from build123d import *

# Parameters (mm, degrees)
SKETCH_1_W      = 20
SKETCH_1_H      = 20
SKETCH_1_R      = 1.6
EXTRUDE_1_DEPTH = 20
FILLET_1_R      = 2


with BuildPart() as part:
    # 草图1 → 凸台-拉伸1 (new body)
    with BuildSketch(Plane(origin=(0, 0, 0), x_dir=(1, 0, 0), z_dir=(0, 1, 0))):
        Rectangle(SKETCH_1_W, SKETCH_1_H)
        Circle(SKETCH_1_R, mode=Mode.SUBTRACT)
    extrude(amount=EXTRUDE_1_DEPTH)

    # 圆角1
    fillet_1_edges = [part.edges().sort_by_distance(p)[0] for p in [
        (10, 10, 10),
        (-10, 10, 10),
        (-10, 10, -10),
        (10, 10, -10),
    ]]
    fillet(fillet_1_edges, radius=FILLET_1_R)


solid = part.part
Can you work these out from the model? Positions are in its coordinate system, mm. Coordinates: 2 decimals unless noted, no trailing zeros. Loops run counter-clockwise (first coordinate to the right, second up) from the corner with the lowest first, then second, coordinate; pieces in that order, holes last. Notation, with made-up numbers: (-24.75, -3) - (-20.75, -3) arc R31 ccw to (-20.75, 29) - close; hole circle Ø8 at (-8, -21). An arc over 180 degrees is marked (long way). Answer as a JSON object with one key per item and string values. Group by question number.
Item 1: If I drill on L1, parallel to Z at x = 0, y = 8.5; L2, parallel to X at y = 9.75, z = 0.5, over which ranges is the centre line in solid material (lowest first)? Write a range as from..to.
Item 2: If we section it at A-A (z = 0): List the corners of the cut face in (x, y) for me, plus the area to 3 significant figures.
Item 3: If we section it at B-B (y = 16.5): List the corners of the cut face in (x, z) for me, plus the area to 3 significant figures.
Item 4: If we mould it in two halves opening along X, with no side actions, what happens to faces 1 (the face through (9.4, 10.14, -9.43)), 2 (the face through (2, 0, 0)), 3 (the face through (-1.27, 9.86, 0.97))? For each: released by +X, released by -X, zero draft, split by the parting line, or undercut.
Item 5: If we section it at C-C (x = 0): List the corners of the cut face in (y, z) for me, plus the area to 3 significant figures.
Returned:
{
 "1": {"L1": "z = -10..-1.6, 1.6..10", "L2": "x = -10..-1.52, 1.52..10"},
 "2": {"outline": "(-10, 0) - (-1.6, 0) - (-1.6, 20) - (-10, 20) - close; (1.6, 0) - (10, 0) - (10, 20) - (1.6, 20) - close", "area": "336 mm²"},
 "3": {"outline": "(-10, -8) arc R2 ccw to (-8, -10) - (8, -10) arc R2 ccw to (10, -8) - (10, 8) arc R2 ccw to (8, 10) - (-8, 10) arc R2 ccw to (-10, 8) - close; hole circle Ø3.2 at (0, 0)", "area": "389 mm²"},
 "4": {"face 1": "released by +X", "face 2": "zero draft", "face 3": "undercut"},
 "5": {"outline": "(0, -10) - (20, -10) - (20, -1.6) - (0, -1.6) - close; (0, 1.6) - (20, 1.6) - (20, 10) - (0, 10) - close", "area": "336 mm²"}
}
